Can you work these out from the model? Positions are in its coordinate system, mm. A direction names the side the tool comes from. Round coordinates to 2 decimals unless told otherwise and drop trailing zeros. Loops run counter-clockwise (first coordinate to the right, second up) from the corner with the lowest first, then second, coordinate; pieces in that order, holes last. Notation, with made-up numbers: M 77.5,70.25 L 119.5,70.25 A23 cw 119.5,103.25 Z; hole C -9,-4 d8. An arc over 180 degrees is marked long. Return JSON: item names as keys, results as strings.
```python
from build123d import *

# Parameters (mm, degrees)
SKETCH1_W           = 78
SKETCH1_H           = 59
SKETCH1_R           = 6.000383827
SKETCH1_W_2         = 6
SKETCH1_H_2         = 6
BOSS_EXTRUDE1_DEPTH = 2


with BuildPart() as part:
    # Sketch1 → Boss-Extrude1 (new body)
    with BuildSketch(Plane.XY):
        Rectangle(SKETCH1_W, SKETCH1_H)
        with Locations((0.71, 5.82)):
            Circle(SKETCH1_R, mode=Mode.SUBTRACT)
        with Locations((-23, 13.5)):
            Rectangle(SKETCH1_W_2, SKETCH1_H_2, mode=Mode.SUBTRACT)
        with Locations((23, 13.5)):
            Rectangle(SKETCH1_W_2, SKETCH1_H_2, mode=Mode.SUBTRACT)
    extrude(amount=-BOSS_EXTRUDE1_DEPTH)


solid = part.part
```
Q1. Suppose I cut it at B-B, the plane z = -1.1. Please give me the cut outline in (x, y), plus the area to 3 significant figures.
Results:
{"outline": "M -39,-29.5 L 39,-29.5 L 39,29.5 L -39,29.5 Z; hole M -26,10.5 L -20,10.5 L -20,16.5 L -26,16.5 Z; hole C 0.71,5.82 d12; hole M 20,10.5 L 26,10.5 L 26,16.5 L 20,16.5 Z", "area": "4,420 mm2"}
Q2. Thinking about a two-plate mould opening in X: for faces 3 (the flat face through (-39, 0, -1)), 4 (the flat face through (39, 0, -1)), 5 (the flat face through (-20, 13, -1)), 6 (the flat face through (-1, -6, 0)), which applies, pulls with the +X half, pulls with the -X half, needs draft (parallel to the pull), parting line crosses it, or undercut?
Results:
{"face 3": "pulls with the -X half", "face 4": "pulls with the +X half", "face 5": "undercut", "face 6": "needs draft"}
Q3. On a 3-axis mill with a long thin cutter (end or side, diameter ignored), from which of +Z, -Z, +X, -X, +Y, -Y can I reach the whole of each face in a straight line? I mean faces 1 (the flat face through (-1, -6, -2)), 2 (the flat face through (-23, 16.5, -1)). Say none if no direction works.
Results:
{"face 1": "-Z, +X, -X, +Y, -Y", "face 2": "+Z, -Z"}
Q4. Suppose I cut it at C-C, the plane y = 5.82. Please give me the cut outline in (x, z), plus the area to 3 significant figures.
Results:
{"outline": "M -39,-2 L -5.29,-2 L -5.29,0 L -39,0 Z; M 6.71,-2 L 39,-2 L 39,0 L 6.71,0 Z", "area": "132 mm2"}
Q5. Suppose I cut it at A-A, the plane x = 23.5. Please give me the cut outline in (y, z).
Results:
{"outline": "M -29.5,-2 L 10.5,-2 L 10.5,0 L -29.5,0 Z; M 16.5,-2 L 29.5,-2 L 29.5,0 L 16.5,0 Z"}
Q6. If I drill on line 1 along X through (y, z) = (13, -0.6); line 2 along Y through (x, z) = (0.71, -1.35); line 3 along X through (y, z) = (1, -1.35), over which ranges is the centre line in solid material (lowest first)?
Results:
{"line 1": "x = -39 to -26, -20 to 20, 26 to 39", "line 2": "y = -29.5 to -0.18, 11.82 to 29.5", "line 3": "x = -39 to -2.86, 4.28 to 39"}
